from build123d import *

# Parameters (mm, degrees)
F0_W     = 520.7
F0_H     = 88.9
F0_R     = 12.7
F1_DEPTH = 19.05


with BuildPart() as f1:
    # F0 (on Top) → F1 (new body)
    with BuildSketch(Plane.XY):
        with Locations((-3001.411803, -2580.956636)):
            Rectangle(F0_W, F0_H)
        with Locations((-3175.321132, -2580.956636)):
            Circle(F0_R, mode=Mode.SUBTRACT)
        with Locations((-3099.121132, -2580.956636)):
            Circle(F0_R, mode=Mode.SUBTRACT)
        with Locations((-3022.921132, -2580.956636)):
            Circle(F0_R, mode=Mode.SUBTRACT)
        with Locations((-2880.046132, -2580.956636)):
            Circle(F0_R, mode=Mode.SUBTRACT)
        with Locations((-2829.246132, -2580.956636)):
            Circle(F0_R, mode=Mode.SUBTRACT)
        with Locations((-2778.446132, -2580.956636)):
            Circle(F0_R, mode=Mode.SUBTRACT)
    extrude(amount=F1_DEPTH)


solid = f1.part
Build history of the part. All positions in model axes, mm. Round coordinates to 2 decimals unless told otherwise and drop trailing zeros. Write each loop counter-clockwise with the first axis right and the second up, starting at its lowest first coordinate (ties: lowest second). Pieces come first, ordered by that corner, then holes. Notation, with made-up numbers: (-35.75, -27.5) - (-16.75, -27.5) arc R27 ccw to (-16.75, 10.5) - close; hole circle Ø2 at (-13.5, -9). An arc over 180 degrees is marked (long way). One line per question, with ' | ' between items.
1. Band-saw the part on A-A, the plane x = -3170.5. Write the cut outline in (y, z), and give its area (3 significant figures).
Results are:
outline: (-2625.41, 0) - (-2592.71, 0) - (-2592.71, 19.05) - (-2625.41, 19.05) - close; (-2569.21, 0) - (-2536.51, 0) - (-2536.51, 19.05) - (-2569.21, 19.05) - close | area: 1,250 mm^2
2. Band-saw the part on B-B, the plane y = -2586. Write the cut outline in (x, z).
Results are:
outline: (-3261.76, 0) - (-3186.98, 0) - (-3186.98, 19.05) - (-3261.76, 19.05) - close; (-3163.67, 0) - (-3110.78, 0) - (-3110.78, 19.05) - (-3163.67, 19.05) - close; (-3087.47, 0) - (-3034.58, 0) - (-3034.58, 19.05) - (-3087.47, 19.05) - close; (-3011.27, 0) - (-2891.7, 0) - (-2891.7, 19.05) - (-3011.27, 19.05) - close; (-2868.39, 0) - (-2840.9, 0) - (-2840.9, 19.05) - (-2868.39, 19.05) - close; (-2817.59, 0) - (-2790.1, 0) - (-2790.1, 19.05) - (-2817.59, 19.05) - close; (-2766.79, 0) - (-2741.06, 0) - (-2741.06, 19.05) - (-2766.79, 19.05) - close
3. Mould opens along X. For faces 1 (the face through (-3169.461, -2592.224, 9.392)), 2 (the face through (-2741.062, -2582, 9)), 3 (the face through (-2882.799, -2593.355, 9.392)), 4 (the face through (-3005, -2625.407, 9)) say: released by +X, released by -X, zero draft, split by the parting line, or undercut.
Results are:
face 1: undercut | face 2: released by +X | face 3: undercut | face 4: zero draft
4. Band-saw the part on C-C, the plane z = 13.75. Write the cut outline in (x, y).
Results are:
outline: (-3261.76, -2625.41) - (-2741.06, -2625.41) - (-2741.06, -2536.51) - (-3261.76, -2536.51) - close; hole circle Ø25.4 at (-3175.32, -2580.96); hole circle Ø25.4 at (-3099.12, -2580.96); hole circle Ø25.4 at (-3022.92, -2580.96); hole circle Ø25.4 at (-2880.05, -2580.96); hole circle Ø25.4 at (-2829.25, -2580.96); hole circle Ø25.4 at (-2778.45, -2580.96)
5. Band-saw the part on D-D, the plane x = -2832. Write the cut outline in (y, z).
Results are:
outline: (-2625.41, 0) - (-2593.35, 0) - (-2593.35, 19.05) - (-2625.41, 19.05) - close; (-2568.56, 0) - (-2536.51, 0) - (-2536.51, 19.05) - (-2568.56, 19.05) - close
6. Drop a flat-ended pin along its axis: pin 1 Ø5 at (x, y) = (-2941, -2609) entering from -Z. Give the stop position or say it passes through.
Results are:
pin 1: z = 0
7. Drill centre lines: line 1 along Y through (x, z) = (-2771, 10.5); line 2 along Y through (x, z) = (-2824, 16.5). Where is each one in solid material? Low to high. Write a range as from..to.
Results are:
line 1: -2625.41..-2591.24, -2570.67..-2536.51 | line 2: -2625.41..-2592.52, -2569.39..-2536.51
